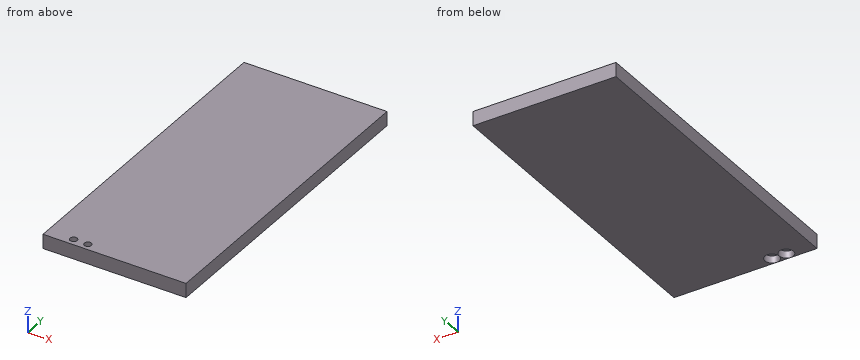
```python
from build123d import *

# Parameters (mm, degrees)
ESQUISSE3_W             = 60
ESQUISSE3_H             = 133
BOSS_EXTRU_2_DEPTH      = 6
ESQUISSE4_R             = 1.5
ENL_V_MAT_EXTRU_1_DEPTH = 74.200068306
ESQUISSE5_R             = 2.995
ENL_V_MAT_EXTRU_2_DEPTH = 3


with BuildPart() as part:
    # Esquisse3 → Boss.-Extru.2 (new body)
    with BuildSketch(Plane.XY):
        Rectangle(ESQUISSE3_W, ESQUISSE3_H)
    extrude(amount=BOSS_EXTRU_2_DEPTH)

    # Esquisse4 → Enlèv. mat.-Extru.1 (cut, through all)
    with BuildSketch(Plane(origin=(0, 0, 0), x_dir=(-1, 0, 0), z_dir=(0, 0, -1))):
        with Locations((13.05, -63.5)):
            Circle(ESQUISSE4_R)
        with Locations((19.05, -63.5)):
            Circle(ESQUISSE4_R)
    extrude(amount=-ENL_V_MAT_EXTRU_1_DEPTH, mode=Mode.SUBTRACT)

    # Esquisse5 → Enlèv. mat.-Extru.2 (cut)
    with BuildSketch(Plane(origin=(0, 0, 0), x_dir=(-1, 0, 0), z_dir=(0, 0, -1))):
        with Locations((13.05, -63.5)):
            Circle(ESQUISSE5_R)
        with Locations((19.05, -63.5)):
            Circle(ESQUISSE5_R)
    extrude(amount=-ENL_V_MAT_EXTRU_2_DEPTH, mode=Mode.SUBTRACT)


solid = part.part
```
Verification items for the finished model (mm, model axes). Round coordinates to 2 decimals unless told otherwise and drop trailing zeros. Write each loop counter-clockwise with the first axis right and the second up, starting at its lowest first coordinate (ties: lowest second). Pieces come first, ordered by that corner, then holes.
1. Section check A-A on x = -13.05. Enter the section's corners in (y, z) (3 decimals), plus the area to 3 significant figures.
2. Gauge pin test, flat ends, axial feed: P1, Ø6, axis at x = 14.5, y = -22.5, coming from the -Z side; P2, Ø5.5, axis at x = -13.05, y = -63.5, coming from the -Z side. Record the tip position at first contact, or that the pin passes through.
3. Section check B-B on y = -63.5. Enter the section's corners in (x, z) (3 decimals), plus the area to 3 significant figures.
4. Scan lines: L1, parallel to Y at x = -13.05, z = 4.6; L2, parallel to Y at x = -17, z = 2.65. Record each from-to range of solid material in increasing order.
Answer:
1. outline: (-66.5, 0) - (-66.495, 0) - (-66.495, 3) - (-65, 3) - (-65, 6) - (-66.5, 6) - close; (-62, 3) - (-60.505, 3) - (-60.505, 0) - (66.5, 0) - (66.5, 6) - (-62, 6) - close
1. area: 771 mm2
2. P1: stops at z = 0
2. P2: stops at z = 3
3. outline: (-30, 0) - (-22.045, 0) - (-22.045, 3) - (-20.55, 3) - (-20.55, 6) - (-30, 6) - close; (-17.55, 3) - (-16.055, 3) - (-16.055, 0) - (-16.045, 0) - (-16.045, 3) - (-14.55, 3) - (-14.55, 6) - (-17.55, 6) - close; (-11.55, 3) - (-10.055, 3) - (-10.055, 0) - (30, 0) - (30, 6) - (-11.55, 6) - close
3. area: 306 mm2
4. L1: y = -66.5 to -65, -62 to 66.5
4. L2: y = -66.5 to -65.68, -61.32 to 66.5
